Design review of the part shown in the three views and the two pictorial views. Dimensions are in mm from the part's minimum x, y and z. Give positions to 0.01 mm unless a question says otherwise; leave off trailing zeros. Order: outer loops, then holes, each group sorted by start corner. A loop starts at its lowest first (then second) coordinate and runs counter-clockwise, first axis right, second up. Notation, with made-up numbers: (75.25, 13.25) - (103.25, 13.25) arc R27 cw to (103.25, 43.25) - close; hole circle Ø1 at (36.5, -21). An arc over 180 degrees is marked (long way). Put each result on its own line as item: value. Start each with the question number.
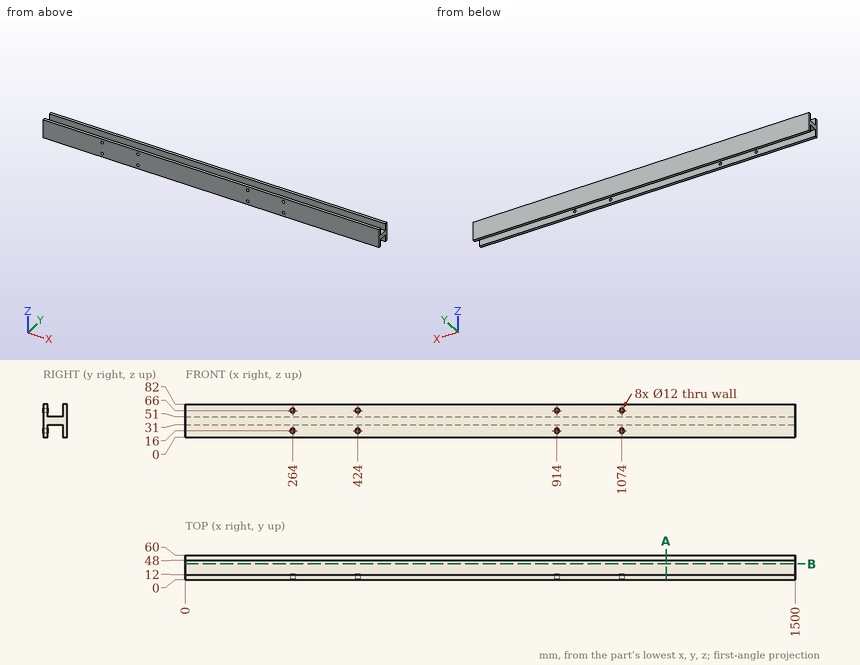
1. Add section A-A, the plane x = 1183. Give the boundary of the cut face in (y, z), then the cut area to 3 significant figures.
2. Wall thickness on line 1 (Z direction, x = 914, y = 4); line 2 (X direction, y = 3.75, z = 16); line 3 (Y direction, x = 247.5, z = 29): over which ranges is each line inside the solid? List them lowest first. Write a range as from..to.
3. Add section B-B, the plane y = 39. Give the boundary of the cut face in (x, z), then the cut area to 3 significant figures.
4. Clearance check with flat-ended pins moving along their axes: pin 1 (1 mm diameter, centred on x = 628.5, y = 15.5, fed in from +Z); pin 2 (7 mm diameter, centred on x = 264, z = 16, fed in from -Y); pin 3 (6 mm diameter, centred on x = 984, y = 39.5, fed in from -Z). State where each tip first meets the part, or that it passes through.
Found:
1. outline: (0, 0) - (12, 0) - (12, 31) - (48, 31) - (48, 0) - (60, 0) - (60, 82) - (48, 82) - (48, 51) - (12, 51) - (12, 82) - (0, 82) - close
1. area: 2,690 mm^2
2. line 1: z = 0..10, 22..60, 72..82
2. line 2: x = 0..258, 270..418, 430..908, 920..1068, 1080..1500
2. line 3: y = 0..12, 48..60
3. outline: (0, 31) - (1500, 31) - (1500, 51) - (0, 51) - close
3. area: 30,000 mm^2
4. pin 1: stops at z = 51
4. pin 2: stops at y = 48
4. pin 3: stops at z = 31
